For this review, take the finished solid that the model builds, in its own axes (mm). A direction names the side the tool comes from. Give positions to 0.01 mm unless a question says otherwise; leave off trailing zeros. Write each loop counter-clockwise with the first axis right and the second up, starting at its lowest first coordinate (ties: lowest second). Pieces come first, ordered by that corner, then holes.
Q1. We need section C-C (x = 2). Write out the cut boundary in (y, z).
Q2. Machinability: for faces 1 (the cylindrical face through (22, -1, 15)), 2 (the flat face through (-23.06, -1.28, -10.83)), 3 (the flat face through (12, 1, -15)), which of the approach directions +Z, -Z, +X, -X, +Y, -Y give a long, thin tool a straight path to every point of the face, cutting with its end or side? Answer none if there is none.
Q3. We need section A-A (y = -0.85). Write out the cut boundary in (x, z).
Q4. Mouldability with a two-part tool opening along X and no side actions: class faces 4 (the flat face through (0, 1, -22)), 5 (the flat face through (0, 1, 19.5)), 6 (the flat face through (-18.8, -1.3, 17)), 7 (the flat face through (-23.041, -1.282, 10.824)) as released by +X, released by -X, zero draft, split by the parting line, or undercut.
Q5. For line 1 (Z direction, x = -7, y = 1.3); line 2 (X direction, y = 1.85, z = 6.5); line 3 (Y direction, x = 15.5, z = 0.5), list the stretches that pass through material, from the lowest coordinate up.
Q6. Insertion check: P1, Ø3, axis at x = -5, z = -17.5, coming from the -Y side; P2, Ø22, axis at x = 7, z = 10, coming from the -Y side; P3, Ø3, axis at y = 1, z = -14, coming from the +X side; P4, Ø3, axis at x = 21.5, y = 1, coming from the -Z side. Each pin has a flat end and moves straight along its axis. Give the tip position at first contact, or say it passes through.
Q7. We need section B-B (z = 3). Write out the cut boundary in (x, y).
Q8. We need section D-D (x = -21). Write out the cut boundary in (y, z), then the cut area to 3 significant figures.
```python
from build123d import *

# Parameters (mm, degrees)
SKETCH1_W           = 8
SKETCH1_H           = 18
SKETCH1_W_2         = 24
SKETCH1_H_2         = 8
BOSS_EXTRUDE1_DEPTH = 2.5
BOSS_EXTRUDE2_DEPTH = 2.6


with BuildPart() as part:
    # Sketch1 → Boss-Extrude1 (new body)
    with BuildSketch(Plane(origin=(0, 0, 0), x_dir=(1, 0, 0), z_dir=(0, 1, 0))):
        with BuildLine():
            Line((-26.5, 8), (-26.5, -8))
            ThreePointArc((-26.5, -8), (-22.399494937, -17.899494937), (-12.5, -22))
            Line((-12.5, -22), (12.5, -22))
            ThreePointArc((12.5, -22), (22.399494937, -17.899494937), (26.5, -8))
            Line((26.5, -8), (26.5, 8))
            ThreePointArc((26.5, 8), (22.399494937, 17.899494937), (12.5, 22))
            Line((12.5, 22), (-12.5, 22))
            ThreePointArc((-12.5, 22), (-22.399494937, 17.899494937), (-26.5, 8))
        make_face()
        with Locations((21, 0)):
            Rectangle(SKETCH1_W, SKETCH1_H, mode=Mode.SUBTRACT)
        with Locations((0, 15.5)):
            Rectangle(SKETCH1_W_2, SKETCH1_H_2, mode=Mode.SUBTRACT)
        with Locations((0, -15.5)):
            Rectangle(SKETCH1_W_2, SKETCH1_H_2, mode=Mode.SUBTRACT)
    extrude(amount=BOSS_EXTRUDE1_DEPTH)

    # Sketch2 → Boss-Extrude2 (add)
    with BuildSketch(Plane.XZ):
        with BuildLine():
            ThreePointArc((18.264443185, -16.232478045), (20.732478045, -13.764443185), (22.207554554, -10.601131403))
            Line((22.207554554, -10.601131403), (23.89792475, -11.054064732))
            ThreePointArc((23.89792475, -11.054064732), (22.165994123, -14.768201949), (19.268201949, -17.665994123))
            Line((19.268201949, -17.665994123), (18.264443185, -16.232478045))
        make_face()
        with BuildLine():
            ThreePointArc((19.268201949, 17.665994123), (22.165994123, 14.768201949), (23.89792475, 11.054064732))
            Line((23.89792475, 11.054064732), (22.207554554, 10.601131403))
            ThreePointArc((22.207554554, 10.601131403), (20.732478045, 13.764443185), (18.264443185, 16.232478045))
            Line((18.264443185, 16.232478045), (19.268201949, 17.665994123))
        make_face()
        with BuildLine():
            Line((-18.264443185, -16.232478045), (-19.268201949, -17.665994123))
            ThreePointArc((-19.268201949, -17.665994123), (-22.165994123, -14.768201949), (-23.89792475, -11.054064732))
            Line((-23.89792475, -11.054064732), (-22.207554554, -10.601131403))
            ThreePointArc((-22.207554554, -10.601131403), (-20.732478045, -13.764443185), (-18.264443185, -16.232478045))
        make_face()
        with BuildLine():
            ThreePointArc((-18.264443185, 16.232478045), (-20.732478045, 13.764443185), (-22.207554554, 10.601131403))
            Line((-22.207554554, 10.601131403), (-23.89792475, 11.054064732))
            ThreePointArc((-23.89792475, 11.054064732), (-22.165994123, 14.768201949), (-19.268201949, 17.665994123))
            Line((-19.268201949, 17.665994123), (-18.264443185, 16.232478045))
        make_face()
    extrude(amount=BOSS_EXTRUDE2_DEPTH)


solid = part.part
```
Computed:
1. outline: (0, -22) - (2.5, -22) - (2.5, -19.5) - (0, -19.5) - close; (0, -11.5) - (2.5, -11.5) - (2.5, 11.5) - (0, 11.5) - close; (0, 19.5) - (2.5, 19.5) - (2.5, 22) - (0, 22) - close
2. face 1: +Z, +X, -Y
2. face 2: -X, -Y
2. face 3: +Y, -Y
3. outline: (-23.9, -11.05) arc R11.8 ccw to (-19.27, -17.67) - (-18.26, -16.23) arc R10.05 cw to (-22.21, -10.6) - close; (-23.9, 11.05) - (-22.21, 10.6) arc R10.05 cw to (-18.26, 16.23) - (-19.27, 17.67) arc R11.8 ccw to start; (18.26, -16.23) - (19.27, -17.67) arc R11.8 ccw to (23.9, -11.05) - (22.21, -10.6) arc R10.05 cw to start; (18.26, 16.23) arc R10.05 cw to (22.21, 10.6) - (23.9, 11.05) arc R11.8 ccw to (19.27, 17.67) - close
4. face 4: zero draft
4. face 5: undercut
4. face 6: undercut
4. face 7: released by -X
5. line 1: z = -22 to -19.5, -11.5 to 11.5, 19.5 to 22
5. line 2: x = -26.5 to 17, 25 to 26.5
5. line 3: y = 0 to 2.5
6. P1: passes through
6. P2: stops at y = 0
6. P3: stops at x = 25.76
6. P4: stops at z = -19.82
7. outline: (-26.5, 0) - (17, 0) - (17, 2.5) - (-26.5, 2.5) - close; (25, 0) - (26.5, 0) - (26.5, 2.5) - (25, 2.5) - close
8. outline: (-2.6, -16.18) - (0, -16.18) - (0, -19.12) - (2.5, -19.12) - (2.5, 19.12) - (0, 19.12) - (0, 16.18) - (-2.6, 16.18) - (-2.6, 13.36) - (0, 13.36) - (0, -13.36) - (-2.6, -13.36) - close
8. area: 110 mm2
